from build123d import *

# Parameters (mm, degrees)
BOSS_EXTRUDE1_DEPTH  = 3
BOSS_EXTRUDE2_DEPTH  = 4
SKETCH5_W            = 4
SKETCH5_H            = 4
BOSS_EXTRUDE3_DEPTH  = 10.5
SKETCH7_R            = 2.4
BOSS_EXTRUDE4_DEPTH  = 3
SKETCH9_R            = 0.8
CUT_EXTRUDE6_DEPTH   = 5
BOSS_EXTRUDE10_DEPTH = 24
CUT_EXTRUDE7_DEPTH   = 23
CUT_EXTRUDE10_START  = -24
SKETCH24_W           = 32.370082298
SKETCH24_H           = 20
CUT_EXTRUDE10_DEPTH  = 133.325180249
CIRPATTERN1_COUNT    = 6
BOSS_EXTRUDE11_DEPTH = 20
CIRPATTERN2_COUNT    = 6


with BuildPart() as part:
    # Sketch1 → Boss-Extrude1 (new body)
    with BuildSketch(Plane(origin=(0, 0, 0), x_dir=(1, 0, 0), z_dir=(0, 1, 0))):
        Polygon((0, 60), (-51.961524227, 30), (-51.961524227, -30), (0, -60), (51.961524227, -30), (51.961524227, 30), align=None)
    extrude(amount=BOSS_EXTRUDE1_DEPTH)

    # Sketch2 → Boss-Extrude2 (add)
    with BuildSketch(Plane(origin=(0, 3, 0), x_dir=(1, 0, 0), z_dir=(0, 1, 0))):
        Polygon((35.667295593, 19.777568136), (44.167295593, 34.5), (40.703193978, 36.5), (34.203193978, 25.241669751), (19.480762114, 33.741669751), (13.938199529, 36.941669751), (20.438199529, 48.2), (16.974097914, 50.2), (8.474097914, 35.477568136), (17.480762114, 30.277568136), align=None)
        Polygon((51.961524227, -17), (51.961524227, -21), (34.961524227, -21), (34.961524227, 0), (34.961524227, 10.4), (51.961524227, 10.4), (51.961524227, 6.4), (38.961524227, 6.4), (38.961524227, 0), (38.961524227, -17), align=None)
        Polygon((11.258330249, -53.5), (7.794228634, -55.5), (-0.705771366, -40.777568136), (17.480762114, -30.277568136), (26.487426313, -25.077568136), (34.987426313, -39.8), (31.523324698, -41.8), (25.023324698, -30.541669751), (19.480762114, -33.741669751), (4.758330249, -42.241669751), align=None)
        Polygon((-40.703193978, -36.5), (-44.167295593, -34.5), (-35.667295593, -19.777568136), (-17.480762114, -30.277568136), (-8.474097914, -35.477568136), (-16.974097914, -50.2), (-20.438199529, -48.2), (-13.938199529, -36.941669751), (-19.480762114, -33.741669751), (-34.203193978, -25.241669751), align=None)
        Polygon((-51.961524227, 17), (-51.961524227, 21), (-34.961524227, 21), (-34.961524227, 0), (-34.961524227, -10.4), (-51.961524227, -10.4), (-51.961524227, -6.4), (-38.961524227, -6.4), (-38.961524227, 0), (-38.961524227, 17), align=None)
        Polygon((-11.258330249, 53.5), (-7.794228634, 55.5), (0.705771366, 40.777568136), (-17.480762114, 30.277568136), (-26.487426313, 25.077568136), (-34.987426313, 39.8), (-31.523324698, 41.8), (-25.023324698, 30.541669751), (-19.480762114, 33.741669751), (-4.758330249, 42.241669751), align=None)
    extrude(amount=BOSS_EXTRUDE2_DEPTH)

    # Sketch5 → Boss-Extrude3 (add)
    with BuildSketch(Plane(origin=(0, 7, 0), x_dir=(1, 0, 0), z_dir=(0, 1, 0))):
        with Locations((36.961524227, -5.3)):
            Rectangle(SKETCH5_W, SKETCH5_H)
        Polygon((14.622878281, -31.927568136), (11.158776666, -33.927568136), (13.158776666, -37.391669751), (16.622878281, -35.391669751), align=None)
        with Locations((-36.961524227, 5.3)):
            Rectangle(SKETCH5_W, SKETCH5_H)
        Polygon((-14.622878281, 31.927568136), (-11.158776666, 33.927568136), (-13.158776666, 37.391669751), (-16.622878281, 35.391669751), align=None)
    extrude(amount=BOSS_EXTRUDE3_DEPTH)

    # Sketch7 → Boss-Extrude4 (add)
    with BuildSketch(Plane.XZ):
        with Locations(Location((22.730762114, 39.370834875, 0), (0, 0, 90))):
            Circle(SKETCH7_R)
        with Locations(Location((45.461524227, 0, 0), (0, 0, 90))):
            Circle(SKETCH7_R)
        with Locations(Location((22.730762114, -39.370834875, 0), (0, 0, 90))):
            Circle(SKETCH7_R)
        with Locations(Location((-22.730762114, -39.370834875, 0), (0, 0, 90))):
            Circle(SKETCH7_R)
        with Locations(Location((-45.461524227, 0, 0), (0, 0, 90))):
            Circle(SKETCH7_R)
        with Locations(Location((-22.730762114, 39.370834875, 0), (0, 0, 90))):
            Circle(SKETCH7_R)
    extrude(amount=BOSS_EXTRUDE4_DEPTH)

    # Sketch9 → Cut-Extrude6 (cut)
    with BuildSketch(Plane(origin=(0, 17.5, 0), x_dir=(1, 0, 0), z_dir=(0, 1, 0))):
        with Locations(Location((-36.961524227, 5.3, 0), (0, 0, 270))):
            Circle(SKETCH9_R)
        with Locations(Location((-13.890827473, 34.659618943, 0), (0, 0, 270))):
            Circle(SKETCH9_R)
        with Locations((23.070696754, 29.359618943)):
            Circle(SKETCH9_R)
        with Locations(Location((36.961524227, -5.3, 0), (0, 0, 270))):
            Circle(SKETCH9_R)
        with Locations(Location((13.890827473, -34.659618943, 0), (0, 0, 270))):
            Circle(SKETCH9_R)
        with Locations((-23.070696754, -29.359618943)):
            Circle(SKETCH9_R)
    extrude(amount=-CUT_EXTRUDE6_DEPTH, mode=Mode.SUBTRACT)

    # Sketch22 → Boss-Extrude10 (add)
    with BuildSketch(Plane.XZ):
        Polygon((-34.948372872, 20.207790041), (-34.974645966, -20.162283708), (-0.026273093, -40.370073749), (34.948372872, -20.207790041), (34.974645966, 20.162283708), (0.026273093, 40.370073749), align=None)
    extrude(amount=BOSS_EXTRUDE10_DEPTH)

    # Sketch23 → Cut-Extrude7 (cut)
    with BuildSketch(Plane(origin=(0, 3, 0), x_dir=(1, 0, 0), z_dir=(0, 1, 0))):
        Polygon((-0.023267149, 35.751272573), (-30.973143841, 17.855486345), (-30.949876692, -17.895786229), (0.023267149, -35.751272573), (30.973143841, -17.855486345), (30.949876692, 17.895786229), align=None)
    extrude(amount=-CUT_EXTRUDE7_DEPTH, mode=Mode.SUBTRACT)

    # Sketch24 → Cut-Extrude10 (cut)
    with BuildSketch(Plane(origin=(34.961509419, 0, -0.022753166), x_dir=(-0.0006508060386860347, 0, -0.9999997882257277), z_dir=(0.9999997882257275, 0, -0.0006508060386860346)).offset(CUT_EXTRUDE10_START)):
        with Locations((0, -10)):
            Rectangle(SKETCH24_W, SKETCH24_H)
    cut_extrude10 = extrude(amount=CUT_EXTRUDE10_DEPTH, mode=Mode.SUBTRACT)

    # CirPattern1: Cut-Extrude10 ×6 about axis
    cirpattern1_axis = Axis((0, 0, 0), (0, 1, 0))
    for i in range(1, CIRPATTERN1_COUNT):
        add(cut_extrude10.rotate(cirpattern1_axis, i * 360 / CIRPATTERN1_COUNT), mode=Mode.SUBTRACT)

    # Sketch25 → Boss-Extrude11 (add)
    with BuildSketch(Plane(origin=(0, -20, 0), x_dir=(1, 0, 0), z_dir=(0, 1, 0))):
        Polygon((15.498205495, -26.803379459), (17.662455038, -25.551970687), (19.66553091, -29.016191283), (15.330894041, -31.518795046), (13.332328936, -28.051970158), align=None)
    boss_extrude11 = extrude(amount=BOSS_EXTRUDE11_DEPTH)

    # CirPattern2: Boss-Extrude11 ×6 about axis
    cirpattern2_axis = Axis((0, 0, 0), (0, 1, 0))
    for i in range(1, CIRPATTERN2_COUNT):
        add(boss_extrude11.rotate(cirpattern2_axis, i * 360 / CIRPATTERN2_COUNT))


solid = part.part
Can you work these out from the model? Positions are in its coordinate system, mm. A direction names the side the tool comes from. Give positions to 0.01 mm unless a question says otherwise; leave off trailing zeros. Loops run counter-clockwise (first coordinate to the right, second up) from the corner with the lowest first, then second, coordinate; pieces in that order, holes last. Notation, with made-up numbers: (-28, -39.5) -> (-8, -39.5) arc R30 cw to (-8, -5.5) -> close; hole circle Ø4 at (64.25, -8.75). An arc over 180 degrees is marked (long way). Return JSON: item names as keys, results as strings.
Q1. For pin 1 Ø4.5 at (x, y) = (-45.5, 5) entering from +Z; pin 2 Ø4.5 at (x, y) = (37.5, 12) entering from -Z; pin 3 Ø7 at (x, z) = (21.5, -38) entering from +Y; pin 4 Ø8 at (x, y) = (-9, -15.5) entering from +Z, each with a flat end and sliding along its axis, tell me the tip position at first contact or that it passes through.
Checks:
{"pin 1": "stops at z = 35.03", "pin 2": "stops at z = 3.3", "pin 3": "stops at y = 3", "pin 4": "passes through"}
Q2. I want a section at A-A, the plane x = -22. List the corners of the cut face in (y, z) for me.
Checks:
{"outline": "(-24, -27.66) -> (-20, -27.66) -> (-20, 27.67) -> (-24, 27.67) -> close; (0, -47.3) -> (3, -47.3) -> (3, -32.29) -> (7, -32.29) -> (7, -27.67) -> (3, -27.67) -> (3, -23.04) -> (0, -23.04) -> close; (0, 23.06) -> (3, 23.06) -> (3, 27.67) -> (7, 27.67) -> (7, 32.29) -> (3, 32.29) -> (3, 47.3) -> (0, 47.3) -> close"}
Q3. I need wall thicknesses on probe 1 along Z at (x, y) = (-22, 1); probe 2 along Y at (x, z) = (36, -23.5); probe 3 along Y at (x, z) = (-23.5, 32.5). Which ranges of each line are inside material? Lowest first, please.
Checks:
{"probe 1": "z = -47.3 to -23.04, 23.06 to 47.3", "probe 2": "y = 0 to 7", "probe 3": "y = 0 to 3"}
Q4. I want a section at B-B, the plane y = -13. Count the separate pieces of the cut face and the enclosed holes in it, then the cut area to 3 significant figures.
Checks:
{"separate pieces": "12", "enclosed holes": "0", "area": "257 mm2"}
Q5. On a 3-axis mill with a long thin cutter (end or side, diameter ignored), from which of +Z, -Z, +X, -X, +Y, -Y can I reach the whole of each face in a straight line? I mean faces 1 (the face through (-37, 12, -7.3)), 2 (the face through (-30.68, 4.97, -32.34)), 3 (the face through (-2.43, -10.14, 36.62)). Say none if no direction works.
Checks:
{"face 1": "-Z, +X, -X, +Y", "face 2": "-X, +Y", "face 3": "-X"}
Q6. We'd pull the mould along Y, two halves only. Please class faces 4 (the face through (2.474, -10.14, 36.612)), 5 (the face through (12.145, 12.176, 35.635)), 6 (the face through (-36, 17.5, -5)): released by +Y, released by -Y, zero draft, split by the parting line, or undercut.
Checks:
{"face 4": "undercut", "face 5": "zero draft", "face 6": "released by +Y"}
Q7. I want a section at C-C, the plane z = -14. List the corners of the cut face in (x, y) for me, then the cut area to 3 significant figures.
Checks:
{"outline": "(-51.96, 0) -> (-30.97, 0) -> (-30.97, 3) -> (-34.96, 3) -> (-34.96, 7) -> (-38.96, 7) -> (-38.96, 3) -> (-51.96, 3) -> close; (-34.97, -24) -> (34.95, -24) -> (34.95, -20) -> (-34.97, -20) -> close; (30.95, 0) -> (51.96, 0) -> (51.96, 3) -> (30.95, 3) -> close", "area": "422 mm2"}
